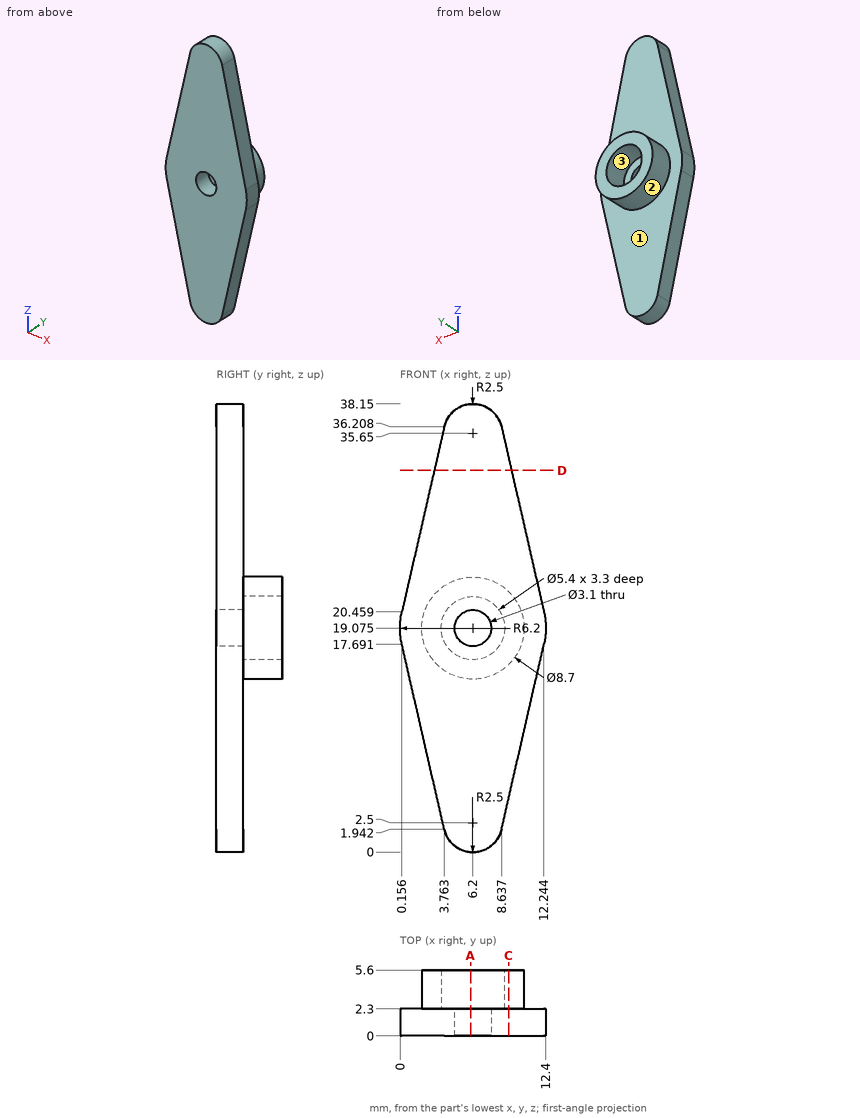
Study the drawing (mm; zero at the part's minimum x, y, z) and answer. Coordinates: 2 decimals unless noted, no trailing zeros. Write each loop counter-clockwise with the first axis right and the second up, starting at its lowest first coordinate (ties: lowest second). Pieces come first, ordered by that corner, then holes. Notation, with made-up numbers: (-40, 51) - (-14, 51) arc R28 cw to (-14, 76) - close; hole circle Ø10 at (52.25, 29.5). An arc over 180 degrees is marked (long way). Answer as a JSON object with one key per item and string values. Group by question number.
1. Each of these flat-tipped pins is pushed along its axis until it touches: P1, Ø2, axis at x = 7.5, y = 2, coming from the +Z side; P2, Ø6, axis at x = 9.5, z = 11, coming from the +Y side. Where does it stop, or does it pass through?
2. A cutting plane is placed at C-C (x = 9.25). Determine the outline of the cut face in (y, z).
3. Consider L1, parallel to Y at x = 7.5, z = 32; L2, parallel to Z at x = 8.5, y = 4.2 (1 decimal); L3, parallel to Z at x = 8, y = 4.1 (1 decimal). Determine where each line is inside the solid, lowest interval first. Write a range as [from, to].
4. A cutting plane is placed at A-A (x = 6). Determine the outline of the cut face in (y, z).
5. A cutting plane is placed at D-D (z = 32.5). Determine the outline of the cut face in (x, y).
6. The mould has two halves that part along Z. Classify the marked faces 1, 2 and 3: +Z half, -Z half, draft (parallel to the pull), parting line (faces both ways), or undercut.
Worked out:
{
 "1": {"P1": "stops at z = 38.13", "P2": "stops at y = 2.3"},
 "2": {"outline": "(0, 4.62) - (2.3, 4.62) - (2.3, 15.97) - (5.6, 15.97) - (5.6, 22.18) - (2.3, 22.18) - (2.3, 33.53) - (0, 33.53) - close"},
 "3": {"L1": "y = [0, 2.3]", "L2": "z = [15.4, 17.7], [20.5, 22.8]", "L3": "z = [15.1, 17.1], [21.1, 23]"},
 "4": {"outline": "(0, 0.01) - (2.3, 0.01) - (2.3, 14.73) - (5.6, 14.73) - (5.6, 16.38) - (2.3, 16.38) - (2.3, 17.54) - (0, 17.54) - close; (0, 20.61) - (2.3, 20.61) - (2.3, 21.77) - (5.6, 21.77) - (5.6, 23.42) - (2.3, 23.42) - (2.3, 38.14) - (0, 38.14) - close"},
 "5": {"outline": "(2.91, 0) - (9.49, 0) - (9.49, 2.3) - (2.91, 2.3) - close"},
 "6": {"face 1": "draft", "face 2": "parting line", "face 3": "undercut"}
}
